from build123d import *

# Parameters (mm, degrees)
F1_DEPTH = 6


with BuildPart() as f1:
    # F0 (on Front) → F1 (new body)
    with BuildSketch(Plane.XZ):
        with BuildLine():
            ThreePointArc((-10.743231, -2.117897), (-9.482978, 5.475), (-3.537462, 10.36286))
            Line((-3.537462, 10.36286), (-7.660854, 12.187504))
            ThreePointArc((-7.660854, 12.187504), (-12.466674, 7.197638), (-14.385115, 0.540742))
            Line((-14.385115, 0.540742), (-10.743231, -2.117897))
        make_face()
        with BuildLine():
            ThreePointArc((-9.482978, -5.475), (-10.251459, -3.848387), (-10.743231, -2.117897))
            Line((-10.743231, -2.117897), (-14.385115, 0.540742))
            Line((-14.385115, 0.540742), (-14.720386, 0.785496))
            Line((-14.720386, 0.785496), (-18.868808, -1.609597))
            Line((-18.868808, -1.609597), (-24.447452, -3.553989))
            Line((-24.447452, -3.553989), (-25.980762, -15))
            Line((-25.980762, -15), (-20.635515, -11.91392))
            Line((-20.635515, -11.91392), (-21.219079, -7.334182))
            Line((-21.219079, -7.334182), (-16.961128, -4.094992))
            Line((-16.961128, -4.094992), (-12.026931, -6.162892))
            Line((-12.026931, -6.162892), (-11.93425, -6.890243))
            Line((-11.93425, -6.890243), (-9.482978, -5.475))
        make_face()
        with BuildLine():
            ThreePointArc((-7.205768, -8.244962), (-8.458531, -6.953831), (-9.482978, -5.475))
            Line((-9.482978, -5.475), (-11.93425, -6.890243))
            Line((-11.93425, -6.890243), (-11.350686, -11.469981))
            Line((-11.350686, -11.469981), (-15.608638, -14.70917))
            Line((-15.608638, -14.70917), (-20.542834, -12.641271))
            Line((-20.542834, -12.641271), (-20.635515, -11.91392))
            Line((-20.635515, -11.91392), (-25.980762, -15))
            Line((-25.980762, -15), (-15.301571, -19.39512))
            Line((-15.301571, -19.39512), (-10.828356, -15.536069))
            Line((-10.828356, -15.536069), (-6.679934, -13.140976))
            Line((-6.679934, -13.140976), (-6.724261, -12.728246))
            Line((-6.724261, -12.728246), (-7.205768, -8.244962))
        make_face()
        with BuildLine():
            Line((6.724261, -12.728246), (7.205768, -8.244962))
            ThreePointArc((7.205768, -8.244962), (0, -10.95), (-7.205768, -8.244962))
            Line((-7.205768, -8.244962), (-6.724261, -12.728246))
            ThreePointArc((-6.724261, -12.728246), (0, -14.395275), (6.724261, -12.728246))
        make_face()
        with BuildLine():
            Line((11.93425, -6.890243), (9.482978, -5.475))
            ThreePointArc((9.482978, -5.475), (8.458531, -6.953831), (7.205768, -8.244962))
            Line((7.205768, -8.244962), (6.724261, -12.728246))
            Line((6.724261, -12.728246), (6.679934, -13.140976))
            Line((6.679934, -13.140976), (10.828356, -15.536069))
            Line((10.828356, -15.536069), (15.301571, -19.39512))
            Line((15.301571, -19.39512), (25.980762, -15))
            Line((25.980762, -15), (20.635515, -11.91392))
            Line((20.635515, -11.91392), (20.542834, -12.641271))
            Line((20.542834, -12.641271), (15.608638, -14.70917))
            Line((15.608638, -14.70917), (11.350686, -11.469981))
            Line((11.350686, -11.469981), (11.93425, -6.890243))
        make_face()
        with BuildLine():
            Line((14.385115, 0.540742), (10.743231, -2.117897))
            ThreePointArc((10.743231, -2.117897), (10.251459, -3.848387), (9.482978, -5.475))
            Line((9.482978, -5.475), (11.93425, -6.890243))
            Line((11.93425, -6.890243), (12.026931, -6.162892))
            Line((12.026931, -6.162892), (16.961128, -4.094992))
            Line((16.961128, -4.094992), (21.219079, -7.334182))
            Line((21.219079, -7.334182), (20.635515, -11.91392))
            Line((20.635515, -11.91392), (25.980762, -15))
            Line((25.980762, -15), (24.447452, -3.553989))
            Line((24.447452, -3.553989), (18.868808, -1.609597))
            Line((18.868808, -1.609597), (14.720386, 0.785496))
            Line((14.720386, 0.785496), (14.385115, 0.540742))
        make_face()
        with BuildLine():
            ThreePointArc((3.537462, 10.36286), (8.906113, 6.370529), (10.95, 0))
            ThreePointArc((10.95, 0), (10.898185, -1.063983), (10.743231, -2.117897))
            Line((10.743231, -2.117897), (14.385115, 0.540742))
            ThreePointArc((14.385115, 0.540742), (12.466674, 7.197638), (7.660854, 12.187504))
            Line((7.660854, 12.187504), (3.537462, 10.36286))
        make_face()
        with BuildLine():
            ThreePointArc((0, 10.95), (1.792929, 10.802218), (3.537462, 10.36286))
            Line((3.537462, 10.36286), (7.660854, 12.187504))
            Line((7.660854, 12.187504), (8.040452, 12.35548))
            Line((8.040452, 12.35548), (8.040452, 17.145665))
            Line((8.040452, 17.145665), (9.145881, 22.949109))
            Line((9.145881, 22.949109), (0, 30))
            Line((0, 30), (0, 23.82784))
            Line((0, 23.82784), (4.257951, 22.043353))
            Line((4.257951, 22.043353), (4.934196, 16.736264))
            Line((4.934196, 16.736264), (0.676245, 13.497074))
            Line((0.676245, 13.497074), (0, 13.780485))
            Line((0, 13.780485), (0, 10.95))
        make_face()
        with BuildLine():
            ThreePointArc((-3.537462, 10.36286), (-1.792929, 10.802218), (0, 10.95))
            Line((0, 10.95), (0, 13.780485))
            Line((0, 13.780485), (-4.257951, 15.564973))
            Line((-4.257951, 15.564973), (-4.934196, 20.872062))
            Line((-4.934196, 20.872062), (-0.676245, 24.111252))
            Line((-0.676245, 24.111252), (0, 23.82784))
            Line((0, 23.82784), (0, 30))
            Line((0, 30), (-9.145881, 22.949109))
            Line((-9.145881, 22.949109), (-8.040452, 17.145665))
            Line((-8.040452, 17.145665), (-8.040452, 12.35548))
            Line((-8.040452, 12.35548), (-7.660854, 12.187504))
            Line((-7.660854, 12.187504), (-3.537462, 10.36286))
        make_face()
    extrude(amount=F1_DEPTH)


solid = f1.part
The listing builds one solid part. Answer for the finished solid, in the listing's coordinates (mm). A direction names the side the tool comes from. Give positions to 0.01 mm unless a question says otherwise; leave off trailing zeros. Write each loop counter-clockwise with the first axis right and the second up, starting at its lowest first coordinate (ties: lowest second). Pieces come first, ordered by that corner, then holes.
1) Find the intervals of material crossed by L1, parallel to X at y = -3, z = -13; L2, parallel to X at y = -4.4, z = -8.5; L3, parallel to X at y = -2.2, z = -10, in increasing order.
2) Given P1, Ø1, axis at y = -3.5, z = 16, coming from the +X side; P2, Ø3, axis at x = -15, z = 9, coming from the +Y side; P3, Ø3, axis at y = -1.5, z = 24.5, coming from the +X side; P4, Ø1, axis at y = -2, z = 1.5, coming from the -X side, each flat-ended and moving along its own axis, determine where each tip first touches the part or whether it passes through.
3) A tool of negligible diameter and unlimited length cuts with its end or side. For faces 4 (the face through (-10.243, -2.958, -3.872)), 5 (the face through (25.225, -2.958, -9.357)), 6 (the face through (8.725, -2.958, -14.322)), from which of +Z, -Z, +X, -X, +Y, -Y can it reach the whole face along a straight path? Write none if from no direction.
4) Section A-A (z = 5.5) is taken. Write down the section's boundary in (x, y).
5) Section D-D (x = -23) is taken. Write down the section's boundary in (y, z).
6) Section B-B (y = -2.1) is taken. Count the separate pieces of the cut face and the enclosed holes in it, and give its area (3 significant figures).
7) Section C-C (z = -1) is taken. Write down the section's boundary in (x, y), and give its area (3 significant figures).
8) For a pull along X with two mould halves and no side action, classify faces 1 (the face through (-2, -6, 11)), 2 (the face through (4.637, -2.958, 26.425)), 3 (the face through (-19.12, -2.958, -5.737)) as pulls with the +X half, pulls with the -X half, needs draft (parallel to the pull), parting line crosses it, or undercut.
Response:
1. L1: x = -25.71 to -19.69, -13.36 to -6.7, -6.18 to 6.18, 6.7 to 13.36, 19.69 to 25.71
1. L2: x = -25.11 to -21.07, -11.73 to -6.9, 6.9 to 11.73, 21.07 to 25.11
1. L3: x = -25.31 to -20.88, -11.54 to -4.46, 4.46 to 11.54, 20.88 to 25.31
2. P1: stops at x = 8.04
2. P2: passes through
2. P3: stops at x = 9.08
2. P4: stops at x = -14.36
3. face 4: +Y, -Y
3. face 5: +Z, +X, +Y, -Y
3. face 6: -Z, +Y, -Y
4. outline: (-13.3, -6) - (-9.47, -6) - (-9.47, 0) - (-13.3, 0) - close; (9.47, -6) - (13.3, -6) - (13.3, 0) - (9.47, 0) - close
5. outline: (-6, -16.23) - (0, -16.23) - (0, -3.05) - (-6, -3.05) - close
6. separate pieces: 1
6. enclosed holes: 4
6. area: 714 mm2
7. outline: (-17.81, -6) - (-10.9, -6) - (-10.9, 0) - (-17.81, 0) - close; (10.9, -6) - (17.81, -6) - (17.81, 0) - (10.9, 0) - close
7. area: 82.9 mm2
8. face 1: needs draft
8. face 2: pulls with the +X half
8. face 3: undercut
